Could you check a few things on this drawing? It's one solid part, dimensions in mm from its lowest x, y, z. Give positions to 0.01 mm unless a question says otherwise; leave off trailing zeros. Loops run counter-clockwise (first coordinate to the right, second up) from the corner with the lowest first, then second, coordinate; pieces in that order, holes last.
1. Imagine slicing it at D-D (x = 7.5). List the corners of the cut face in (y, z) for me.
2. I need wall thicknesses on line 1 along Y through (x, z) = (22.5, 0.8); line 2 along Y through (x, z) = (14, 1.55); line 3 along X through (y, z) = (6.5, 0.55). Which ranges of each line are inside material? Lowest first, please.
3. Imagine slicing it at B-B (x = 22.5). List the corners of the cut face in (y, z) for me.
4. For P1, Ø2, axis at x = 46, y = 32, coming from the -Z side, with a flat end and sliding along its axis, tell me the tip position at first contact or that it passes through.
5. Imagine slicing it at C-C (z = 0.3). Count the separate pieces of the cut face and the enclosed holes in it, plus the area to 3 significant figures.
6. Imagine slicing it at A-A (y = 25). List the corners of the cut face in (x, z) for me.
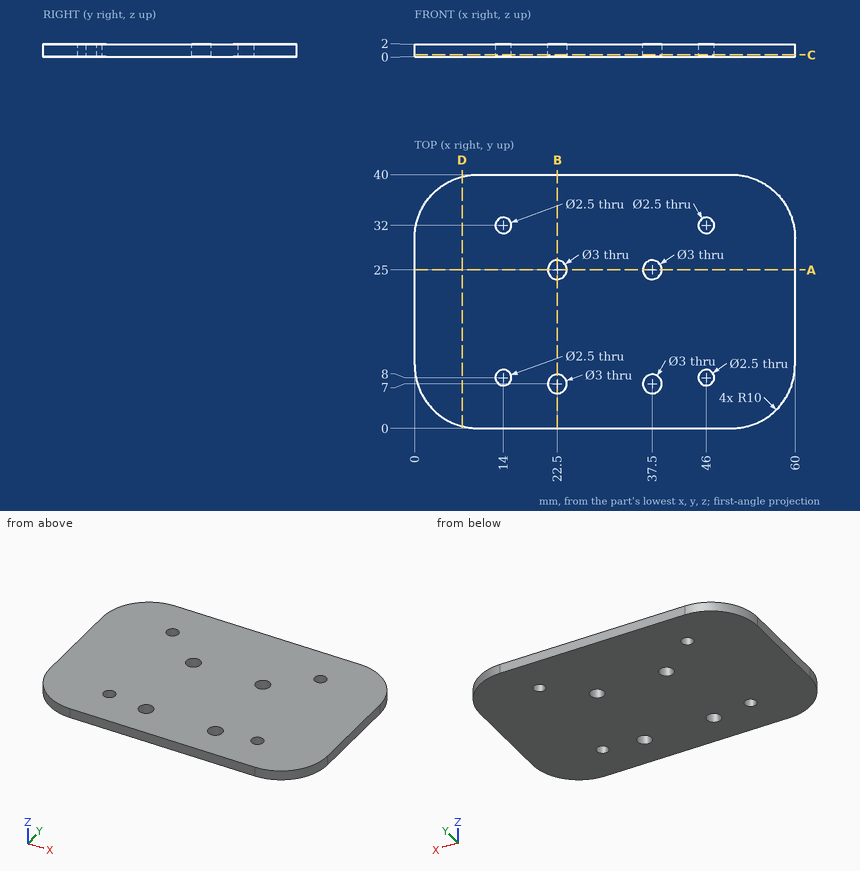
Derived:
1. outline: (0.32, 0) - (39.68, 0) - (39.68, 2) - (0.32, 2) - close
2. line 1: y = 0 to 5.5, 8.5 to 23.5, 26.5 to 40
2. line 2: y = 0 to 6.75, 9.25 to 30.75, 33.25 to 40
2. line 3: x = 0.63 to 21.09, 23.91 to 36.09, 38.91 to 59.37
3. outline: (0, 0) - (5.5, 0) - (5.5, 2) - (0, 2) - close; (8.5, 0) - (23.5, 0) - (23.5, 2) - (8.5, 2) - close; (26.5, 0) - (40, 0) - (40, 2) - (26.5, 2) - close
4. P1: passes through
5. separate pieces: 1
5. enclosed holes: 8
5. area: 2,270 mm2
6. outline: (0, 0) - (21, 0) - (21, 2) - (0, 2) - close; (24, 0) - (36, 0) - (36, 2) - (24, 2) - close; (39, 0) - (60, 0) - (60, 2) - (39, 2) - close
